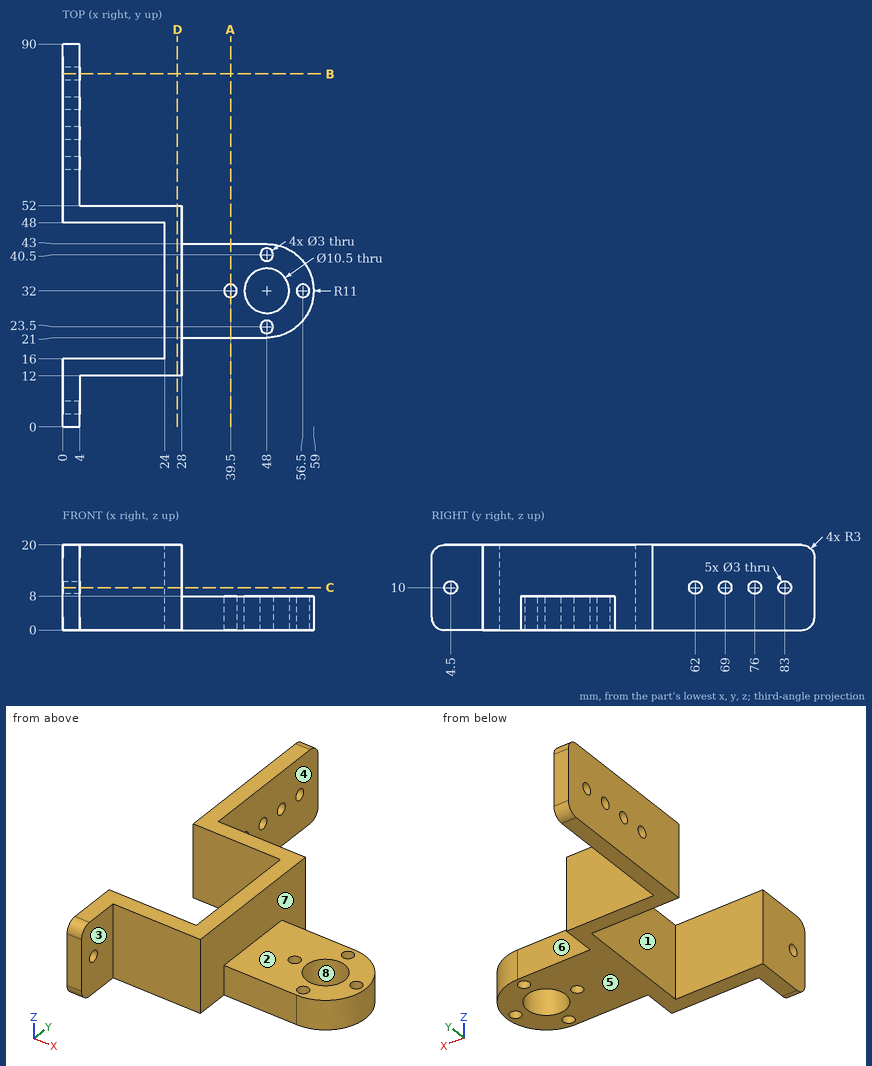
Can you work these out from the drawing? Everything is in mm from the part's minimum corner. A direction names the side the tool comes from. Round coordinates to 2 decimals unless told otherwise and drop trailing zeros. Loops run counter-clockwise (first coordinate to the right, second up) from the corner with the lowest first, then second, coordinate; pieces in that order, holes last. Notation, with made-up numbers: (-1.75, 73.5) -> (35.25, 73.5) arc R37 ccw to (35.25, 111.5) -> close; hole circle Ø2 at (46.25, 21.5). An arc over 180 degrees is marked (long way). Answer in a Markdown table with one row per item.
Item 1: On a 3-axis mill with a long thin cutter (end or side, diameter ignored), from which of +Z, -Z, +X, -X, +Y, -Y can I reach the whole of each face in a straight line? I mean the marked faces 1, 2, 3, 4 and 5. Say none if no direction works.
Answer block:
| item | result |
|---|---|
| face 1 | +Z, -Z, -X |
| face 2 | +Z, +X, +Y, -Y |
| face 3 | +Z, -Z, +X, -Y |
| face 4 | +Z, -Z, +X, +Y |
| face 5 | -Z, +X, -X, +Y, -Y |
Item 2: Suppose I cut it at C-C, the plane z = 10. Give the number of separate pieces and of enclosed holes in the cut face, plus the area to 3 significant figures.
Answer block:
| item | result |
|---|---|
| separate pieces | 6 |
| enclosed holes | 0 |
| area | 492 mm² |
Item 3: Suppose I cut it at A-A, the plane x = 39.5. List the corners of the cut face in (y, z) for me, plus the area to 3 significant figures.
Answer block:
| item | result |
|---|---|
| outline | (21, 0) -> (30.5, 0) -> (30.5, 8) -> (21, 8) -> close; (33.5, 0) -> (43, 0) -> (43, 8) -> (33.5, 8) -> close |
| area | 152 mm² |
Item 4: Will these pins go through, and if not, where does the flat tip stop? P1, Ø2, axis at y = 79.5, z = 17.5, coming from the -X side; P2, Ø2, axis at y = 40.5, z = 12, coming from the -X side; P3, Ø10, axis at y = 73.5, z = 8, coming from the +X side; P4, Ø1.8, axis at x = 56.5, y = 32, coming from the -Z side.
Answer block:
| item | result |
|---|---|
| P1 | x = 0 |
| P2 | x = 24 |
| P3 | x = 4 |
| P4 | through |
Item 5: If I drill on probe 1 along Z at (x, y) = (1.5, 69); probe 2 along Y at (x, z) = (39.5, 3.5); probe 3 along Y at (x, z) = (22.5, 16), over which ranges is the centre line in solid material (lowest first)?
Answer block:
| item | result |
|---|---|
| probe 1 | 0 to 8.5, 11.5 to 20 |
| probe 2 | 21 to 30.5, 33.5 to 43 |
| probe 3 | 12 to 16, 48 to 52 |
Item 6: Suppose I cut it at B-B, the plane y = 83. List the corners of the cut face in (x, z) for me.
Answer block:
| item | result |
|---|---|
| outline | (0, 0) -> (4, 0) -> (4, 8.5) -> (0, 8.5) -> close; (0, 11.5) -> (4, 11.5) -> (4, 20) -> (0, 20) -> close |
Item 7: Suppose I cut it at D-D, the plane x = 27. List the corners of the cut face in (y, z) for me.
Answer block:
| item | result |
|---|---|
| outline | (12, 0) -> (52, 0) -> (52, 20) -> (12, 20) -> close |
Item 8: We'd pull the mould along Y, two halves only. Please class the marked faces 6, 7 and 8: released by +Y, released by -Y, zero draft, split by the parting line, or undercut.
Answer block:
| item | result |
|---|---|
| face 6 | released by +Y |
| face 7 | zero draft |
| face 8 | undercut |
